Geometry: final body of the model. Coordinates: model frame, mm. Face numbers are marked on the shaded views. A direction names the side the tool comes from. Round coordinates to 2 decimals unless told otherwise and drop trailing zeros. Loops run counter-clockwise (first coordinate to the right, second up) from the corner with the lowest first, then second, coordinate; pieces in that order, holes last. Notation, with made-up numbers: (53.5, -37) - (71.5, -37) arc R26 ccw to (71.5, -16) - close; hole circle Ø5 at (-4.5, 75). An arc over 180 degrees is marked (long way). Write item = value, one per line. Start each with the question number.
Item 1: Line query: line 1 (Y direction, x = 298.5, z = 226.5); line 2 (X direction, y = -602.5, z = 1005); line 3 (X direction, y = -173, z = 263). Output: solid intervals per line, ascending. Write a range as from..to.
Item 2: Section A-A (y = -678.5). Return loops of the section in (x, z).
Item 3: Draft query along Y for the marked faces 4, 5 and 6. Return one class per face: pulls with the +Y half, pulls with the -Y half, needs draft (parallel to the pull), parting line crosses it, or undercut.
Item 4: Access query for the marked faces 1, 2 and 3. Directions: +Z, -Z, +X, -X, +Y, -Y. A direction counts if a zero-diameter tool reaches every point of the face in a straight line with its end or side. Return the directions, or none.
Item 5: First-contact query: pin 1 (8 mm diameter, centred on x = 617, z = 943.5, fed in from -Y); pin 2 (4 mm diameter, centred on y = -852, z = 1052.5, fed in from -X); pin 3 (1.5 mm diameter, centred on x = 859, z = 500.5, fed in from +Y). Flat tips, straight axial feed; report the tip coordinate or a pass-through.
Item 6: Section B-B (y = -877). Return loops of the section in (x, z), plus the area to 3 significant figures.
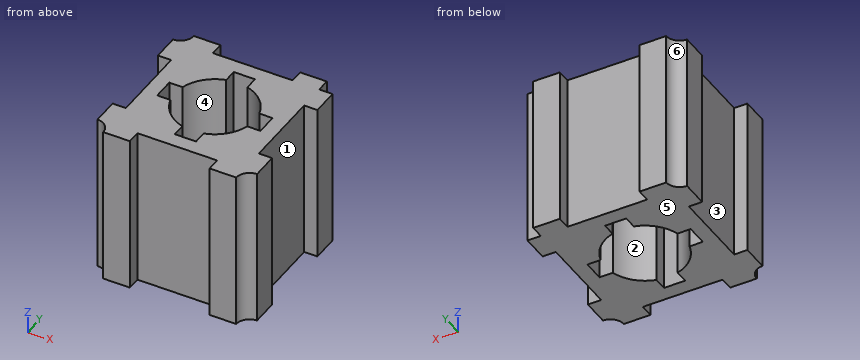
from build123d import *

# Parameters (mm, degrees)
F1_DEPTH = 1524


with BuildPart() as f1:
    # F0 (on Top) → F1 (new body)
    with BuildSketch(Plane.XY):
        with BuildLine():
            ThreePointArc((127, 127), (89.802561, 37.197439), (0, 0))
            Line((0, 0), (0, -254))
            Line((0, -254), (127, -254))
            Line((127, -254), (127, -635))
            Line((127, -635), (127, -1016))
            Line((127, -1016), (0, -1016))
            Line((0, -1016), (0, -1270))
            ThreePointArc((0, -1270), (89.802561, -1307.197439), (127, -1397))
            Line((127, -1397), (381, -1397))
            Line((381, -1397), (381, -1270))
            Line((381, -1270), (1143, -1270))
            Line((1143, -1270), (1143, -1397))
            Line((1143, -1397), (1397, -1397))
            ThreePointArc((1397, -1397), (1434.197439, -1307.197439), (1524, -1270))
            Line((1524, -1270), (1524, -1016))
            Line((1524, -1016), (1397, -1016))
            Line((1397, -1016), (1397, -635))
            Line((1397, -635), (1397, -254))
            Line((1397, -254), (1524, -254))
            Line((1524, -254), (1524, 0))
            Line((1524, 0), (1397, 0))
            Line((1397, 0), (1397, 127))
            Line((1397, 127), (1143, 127))
            Line((1143, 127), (1143, 0))
            Line((1143, 0), (381, 0))
            Line((381, 0), (381, 127))
            Line((381, 127), (127, 127))
        make_face()
        with BuildLine():
            Line((267.017298, -735.520426), (267.017298, -635))
            Line((267.017298, -635), (267.017298, -532.320426))
            Line((267.017298, -532.320426), (394.017298, -532.320426))
            ThreePointArc((394.017298, -532.320426), (492.305962, -364.801425), (660.4, -267.499464))
            Line((660.4, -267.499464), (660.4, -141.096872))
            Line((660.4, -141.096872), (762, -141.096872))
            Line((762, -141.096872), (863.6, -141.096872))
            Line((863.6, -141.096872), (863.6, -268.096872))
            ThreePointArc((863.6, -268.096872), (1031.119001, -366.385537), (1128.420962, -534.479574))
            Line((1128.420962, -534.479574), (1254.823553, -534.479574))
            Line((1254.823553, -534.479574), (1254.823553, -737.679574))
            Line((1254.823553, -737.679574), (1127.823553, -737.679574))
            ThreePointArc((1127.823553, -737.679574), (1029.534889, -905.198575), (861.440851, -1002.500536))
            Line((861.440851, -1002.500536), (861.440851, -1128.903128))
            Line((861.440851, -1128.903128), (658.240851, -1128.903128))
            Line((658.240851, -1128.903128), (658.240851, -1001.903128))
            ThreePointArc((658.240851, -1001.903128), (490.72185, -903.614463), (393.41989, -735.520426))
            Line((393.41989, -735.520426), (267.017298, -735.520426))
        make_face(mode=Mode.SUBTRACT)
    extrude(amount=F1_DEPTH)


solid = f1.part
Taken from the geometry:
q1.line_1 = -1397..-735.52, -532.32..127
q1.line_2 = 127..267.02, 1254.82..1397
q1.line_3 = 0..660.4, 863.6..1524
q2.outline = (127, 0) - (267.02, 0) - (267.02, 1524) - (127, 1524) - close; (1254.82, 0) - (1397, 0) - (1397, 1524) - (1254.82, 1524) - close
q3.face_4 = undercut
q3.face_5 = needs draft
q3.face_6 = pulls with the +Y half
q4.face_1 = +Z, -Z, +X
q4.face_2 = +Z, -Z
q4.face_3 = +Z, -Z, -X
q5.pin_1 = -1270
q5.pin_2 = 127
q5.pin_3 = 0
q6.outline = (127, 0) - (466.65, 0) - (466.65, 1524) - (127, 1524) - close; (1055.19, 0) - (1397, 0) - (1397, 1524) - (1055.19, 1524) - close
q6.area = 1,040,000 mm^2
